Autodesk Inventor part; units mm, degrees
ref_plane "YZ Plane" through (0, 0, 0) normal (1, 0, 0) x (0, 1, 0)
ref_plane "XZ Plane" through (0, 0, 0) normal (0, 1, 0) x (-1, 0, 0)
ref_plane "XY Plane" through (0, 0, 0) normal (0, 0, 1) x (1, 0, 0)
sketch "Sketch1" plane through (0, 0, 0) normal (0, 1, 0) x (-1, 0, 0)
  circle A0 centre (0, 0) radius 120.65
  dimension "d0" = 241.3
sketch "Sketch2" plane through (0, 0, 0) normal (0, 1, 0) x (-1, 0, 0)
  circle A0 centre (0, 0) radius 5.5202
extrude "Extrusion1" add sketch "Sketch2" along normal blind 395.2875
sketch "Sketch3" plane through (0, 395.2875, 0) normal (0, 1, 0) x (1, 0, 0)
  circle A0 centre (0, 0) radius 5.5202
  circle A1 centre (0, 0) radius 165.1
  dimension "d3" = 330.2
loft "Loft1" add profiles "Sketch1", "Sketch3" contours all / A0 | A1
shell "Shell1" thickness 12.7 removed faces 1 at (-20.3699, 395.2875, -51.1247)
properties part number "Trash Can Bottom" material "Polypropylene"
Geometry check sheet. Reference: the model listing, model coordinates, mm. A direction names the side the tool comes from. Give positions to 0.01 mm unless a question says otherwise; leave off trailing zeros. Write each loop counter-clockwise with the first axis right and the second up, starting at its lowest first coordinate (ties: lowest second). Pieces come first, ordered by that corner, then holes. Notation, with made-up numbers: M 48.25,30.5 L 95.25,30.5 A21 ccw 95.25,38.5 Z; hole C 49.5,-18.5 d7. An arc over 180 degrees is marked long. Answer as CSV lines item,"result". Start each with the question number.
Q1. Material ranges on L1, parallel to Y at x = 37, z = -58.5; L2, parallel to X at y = 41, z = 65; L3, parallel to X at y = 208.5, z = 6, recorded low to high.
Q2. Section check B-B, the plane y = 368.5. Record the cut outline in (x, z).
Q3. Section check A-A, the plane x = 0. Record the cut outline in (y, z).
Q4. Go/stop test with flat-tipped pins: pin 1 (1 mm diameter, centred on x = -66.5, y = 140, fed in from -Z); pin 2 (12 mm diameter, centred on x = 65.5, y = 80, fed in from +Z); pin 3 (8 mm diameter, centred on x = 41, z = 80.5, fed in from +Y). Record where each tip stops, or that it passes through.
Q5. Release check for a two-part mould opening along X. For faces 1 (the face through (31.04, 200.41, -139.78)), 2 (the face through (2, 0, 2)), 3 (the face through (130.983, 206.672, 5.765)) record: pulls with the +X half, pulls with the -X half, needs draft (parallel to the pull), parting line crosses it, or undercut.
Q6. Tool access check on faces 4 (the face through (2, 12.7, 2)), 5 (the face through (48, 395.288, 146)). Record the directions out of +Z, -Z, +X, -X, +Y, -Y that give a thin tool (end or side, any length) a straight path to the whole face; none if there is none.
Q7. Section check C-C, the plane y = 124. Record the cut outline in (x, z), then the cut area to 3 significant figures.
Geometry says:
1,L1,"0 to 12.7"
1,L2,"-107.08 to -91.8, 91.8 to 107.08"
1,L3,"-143.97 to -131.18, 131.18 to 143.97"
2,outline,"C 0,0 d324.18; hole C 0,0 d298.62"
3,outline,"M 0,-120.65 L 395.29,-165.1 L 395.29,-152.32 L 12.7,-109.3 L 12.7,109.3 L 395.29,152.32 L 395.29,165.1 L 0,120.65 Z"
4,pin 1,"z = -119.37"
4,pin 2,"z = 115.28"
4,pin 3,"y = 12.7"
5,face 1,"parting line crosses it"
5,face 2,"needs draft"
5,face 3,"undercut"
6,face 4,"+Y"
6,face 5,"+Z, -Z, +X, -X, +Y"
7,outline,"C 0,0 d269.19; hole C 0,0 d243.63"
7,area,"10,300 mm^2"
